Design review of the part built by this model. Coordinates are the model's own, in mm. Face numbers are marked on the shaded views. Coordinates: 2 decimals unless noted, no trailing zeros. Loops run counter-clockwise (first coordinate to the right, second up) from the corner with the lowest first, then second, coordinate; pieces in that order, holes last.
Q1. Wall thickness on probe 1 along Z at (x, y) = (-5.5, 4.5); probe 2 along X at (y, z) = (-1, 3.25); probe 3 along Y at (x, z) = (14.5, 3.25): over which ranges is each line inside the solid? List them lowest first.
Q2. Add section B-B on y = 0. Give the boundary of the cut face in (x, z), and give its area (3 significant figures).
Q3. Add section D-D on x = 17.5. Give the boundary of the cut face in (y, z), and give its area (3 significant figures).
Q4. For P1, Ø3.5, axis at x = 14.5, y = -2, coming from the +Z side; P2, Ø2, axis at x = 12.5, y = -4.5, coming from the -Z side, all flat-tipped, find the tip position at first contact; note any pin that passes through.
Q5. Add section C-C on y = -5.25. Give the boundary of the cut face in (x, z).
Q6. Add section A-A on x = 1. Give the boundary of the cut face in (y, z), and give its area (3 significant figures).
Q7. Draft analysis for pull direction X (two halves, no side actions). For the marked faces 1, 2 and 3, state which applies: released by +X, released by -X, zero draft, split by the parting line, or undercut.
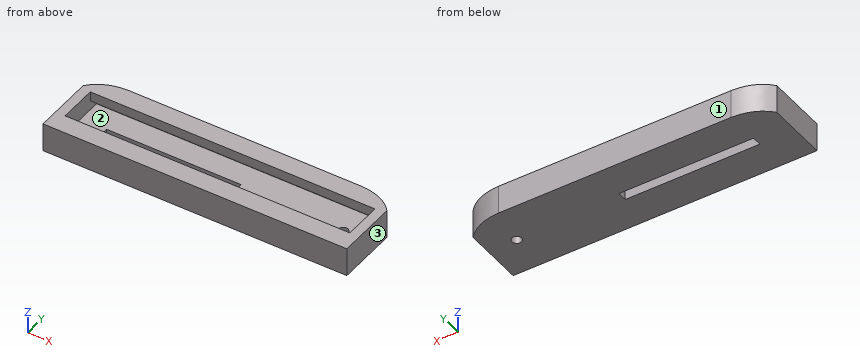
```python
from build123d import *

# Parameters (mm, degrees)
SKETCH1_W           = 63.5
SKETCH1_H           = 16
BOSS_EXTRUDE1_DEPTH = 2
SKETCH2_W           = 63.5
SKETCH2_H           = 16
SKETCH2_W_2         = 59.5
SKETCH2_H_2         = 12
BOSS_EXTRUDE2_DEPTH = 2
SKETCH4_W           = 63.5
SKETCH4_H           = 16
SKETCH4_W_2         = 59.5
SKETCH4_H_2         = 8
BOSS_EXTRUDE3_DEPTH = 2
SKETCH6_R           = 1
CUT_EXTRUDE2_DEPTH  = 33.985792396
SKETCH7_W           = 28.15
SKETCH7_H           = 2
CUT_EXTRUDE3_DEPTH  = 34.287572756
CUT_EXTRUDE4_DEPTH  = 34.287572756


with BuildPart() as part:
    # Sketch1 → Boss-Extrude1 (new body)
    with BuildSketch(Plane.XY):
        Rectangle(SKETCH1_W, SKETCH1_H)
    extrude(amount=BOSS_EXTRUDE1_DEPTH)

    # Sketch2 → Boss-Extrude2 (add)
    with BuildSketch(Plane.XY.offset(2)):
        Rectangle(SKETCH2_W, SKETCH2_H)
        Rectangle(SKETCH2_W_2, SKETCH2_H_2, mode=Mode.SUBTRACT)
    extrude(amount=BOSS_EXTRUDE2_DEPTH)

    # Sketch4 → Boss-Extrude3 (add)
    with BuildSketch(Plane.XY.offset(4)):
        Rectangle(SKETCH4_W, SKETCH4_H)
        Rectangle(SKETCH4_W_2, SKETCH4_H_2, mode=Mode.SUBTRACT)
    extrude(amount=BOSS_EXTRUDE3_DEPTH)

    # Sketch6 → Cut-Extrude2 (cut, through all)
    with BuildSketch(Plane.XY.offset(2)):
        with Locations((25.75, 0)):
            Circle(SKETCH6_R)
    extrude(amount=-CUT_EXTRUDE2_DEPTH, mode=Mode.SUBTRACT)

    # Sketch7 → Cut-Extrude3 (cut, through all)
    with BuildSketch(Plane(origin=(0, 0, 0), x_dir=(-1, 0, 0), z_dir=(0, 0, -1))):
        with Locations((10.325, 0)):
            Rectangle(SKETCH7_W, SKETCH7_H)
    extrude(amount=-CUT_EXTRUDE3_DEPTH, mode=Mode.SUBTRACT)

    # Sketch8 → Cut-Extrude4 (cut, through all)
    with BuildSketch(Plane(origin=(0, 0, 0), x_dir=(-1, 0, 0), z_dir=(0, 0, -1))):
        with BuildLine():
            add(Edge.make_bspline(
                [(24.340057871, 8), (29.079374102, 7.859454073), (31.75, 4.777235297)],
                knots=[0.087220719, 0.087220719, 0.087220719, 1, 1, 1], degree=2))
            Line((31.75, 4.777235297), (31.75, 8))
            Line((31.75, 8), (24.340057871, 8))
        make_face()
    cut_extrude4 = extrude(amount=-CUT_EXTRUDE4_DEPTH, mode=Mode.SUBTRACT)

    # Mirror1: Cut-Extrude4 across plane
    add(cut_extrude4.mirror(Plane(origin=(0, 0, 0), x_dir=(0, 0, 1), z_dir=(1, 0, 0))), mode=Mode.SUBTRACT)


solid = part.part
```
Entries:
1. probe 1: z = 0 to 2, 4 to 6
1. probe 2: x = -31.75 to -29.75, 29.75 to 31.75
1. probe 3: y = -8 to -6, 6 to 8
2. outline: (-31.75, 0) - (-24.4, 0) - (-24.4, 2) - (-29.75, 2) - (-29.75, 6) - (-31.75, 6) - close; (3.75, 0) - (24.75, 0) - (24.75, 2) - (3.75, 2) - close; (26.75, 0) - (31.75, 0) - (31.75, 6) - (29.75, 6) - (29.75, 2) - (26.75, 2) - close
2. area: 82.7 mm2
3. outline: (-8, 0) - (8, 0) - (8, 6) - (4, 6) - (4, 4) - (6, 4) - (6, 2) - (-6, 2) - (-6, 4) - (-4, 4) - (-4, 6) - (-8, 6) - close
3. area: 56.0 mm2
4. P1: stops at z = 2
4. P2: stops at z = 0
5. outline: (-31.75, 0) - (31.75, 0) - (31.75, 6) - (-31.75, 6) - close; hole (-29.75, 2) - (29.75, 2) - (29.75, 4) - (-29.75, 4) - close
6. outline: (-8, 0) - (-1, 0) - (-1, 2) - (-6, 2) - (-6, 4) - (-4, 4) - (-4, 6) - (-8, 6) - close; (1, 0) - (8, 0) - (8, 6) - (4, 6) - (4, 4) - (6, 4) - (6, 2) - (1, 2) - close
6. area: 52.0 mm2
7. face 1: zero draft
7. face 2: undercut
7. face 3: released by +X
